from build123d import *
from OCP.BRepFilletAPI import BRepFilletAPI_MakeChamfer

# Parameters (mm, degrees)
SKETCH1_W           = 16
SKETCH1_H           = 16
BOSS_EXTRUDE1_DEPTH = 25
CIRPATTERN1_COUNT   = 5
CIRPATTERN1_ANGLE   = 160
CHAMFER1_SIZE       = 15
CHAMFER1_SIZE2      = 8.660254038
CHAMFER3_SIZE       = 10
CHAMFER3_SIZE_2     = 5.773502692


with BuildPart() as part:
    # Sketch1 → Boss-Extrude1 (new body)
    with BuildSketch(Plane.XY):
        with BuildLine():
            Line((-150, 0), (0, 0))
            ThreePointArc((0, 0), (-75, -75), (-150, 0))
        make_face()
        with Locations((-55.5, -23)):
            Rectangle(SKETCH1_W, SKETCH1_H, mode=Mode.SUBTRACT)
        with Locations((-94.5, -23)):
            Rectangle(SKETCH1_W, SKETCH1_H, mode=Mode.SUBTRACT)
    extrude(amount=BOSS_EXTRUDE1_DEPTH)

    # Sketch4 → Ø4.0mm Dowel Hole2 (revolve, cut)
    with BuildSketch(Plane(origin=(-1.139418524, -13.023613325, 12.5), x_dir=(0.17364817766693047, 0.9848077530122081, 0), z_dir=(0, 0, 1))):
        Polygon((0, 0), (0, 17.201721238), (2, 16), (2, 0.025), (2.025, 0), align=None)
    f_4_0mm_dowel_hole2 = revolve(axis=Axis((5.114110708, -14.126279253, 12.5), (-0.9848077530122081, 0.17364817766693044, 0)), mode=Mode.SUBTRACT)

    # CirPattern1: Ø4.0mm Dowel Hole2 ×5 about axis
    cirpattern1_axis = Axis((-75, 0, 0), (0, 0, -1))
    for i in range(1, CIRPATTERN1_COUNT):
        add(f_4_0mm_dowel_hole2.rotate(cirpattern1_axis, i * CIRPATTERN1_ANGLE / (CIRPATTERN1_COUNT - 1)), mode=Mode.SUBTRACT)

    # Chamfer1: one chamfer whose edges measure the first distance from different faces: ONE call of the kernel's chamfer builder (chamfer() names one face for all edges)
    chamfer1_edges_1 = [part.edges().sort_by_distance(p)[0] for p in [
        (-55.5, -15, 0),
    ]]
    chamfer1_side_1 = [part.faces().sort_by_distance(p)[0] for p in [
        (-55.5, -15, 12.5),
    ]]
    chamfer1_edges_2 = [part.edges().sort_by_distance(p)[0] for p in [
        (-94.5, -15, 0),
    ]]
    chamfer1_side_2 = [part.faces().sort_by_distance(p)[0] for p in [
        (-94.5, -15, 12.5),
    ]]
    chamfer1 = BRepFilletAPI_MakeChamfer(part.part.solid().wrapped)
    for e in chamfer1_edges_1:
        chamfer1.Add(CHAMFER1_SIZE, CHAMFER1_SIZE2, e.wrapped, chamfer1_side_1[0].wrapped)  # the first distance lies on this face
    for e in chamfer1_edges_2:
        chamfer1.Add(CHAMFER1_SIZE, CHAMFER1_SIZE2, e.wrapped, chamfer1_side_2[0].wrapped)  # the first distance lies on this face
    add(Compound.cast(chamfer1.Shape()), mode=Mode.REPLACE)

    # Chamfer3
    chamfer3_edges_1 = [part.edges().sort_by_distance(p)[0] for p in [
        (-102.5, -23, 25),
    ]]
    chamfer3_side_1 = [part.faces().sort_by_distance(p)[0] for p in [
        (-102.5, -23, 24.884529946),
    ]]
    chamfer3_edges_2 = [part.edges().sort_by_distance(p)[0] for p in [
        (-94.5, -15, 25),
    ]]
    chamfer3_side_2 = [part.faces().sort_by_distance(p)[0] for p in [
        (-94.5, -14.884529946, 25),
    ]]
    chamfer3_edges_3 = [part.edges().sort_by_distance(p)[0] for p in [
        (-86.5, -23, 25),
    ]]
    chamfer3_side_3 = [part.faces().sort_by_distance(p)[0] for p in [
        (-86.5, -23, 24.884529946),
    ]]
    chamfer3_edges_4 = [part.edges().sort_by_distance(p)[0] for p in [
        (-47.5, -23, 25),
    ]]
    chamfer3_side_4 = [part.faces().sort_by_distance(p)[0] for p in [
        (-47.5, -23, 24.884529946),
    ]]
    chamfer3_edges_5 = [part.edges().sort_by_distance(p)[0] for p in [
        (-55.5, -15, 25),
    ]]
    chamfer3_side_5 = [part.faces().sort_by_distance(p)[0] for p in [
        (-55.5, -15, 24.884529946),
    ]]
    chamfer3_edges_6 = [part.edges().sort_by_distance(p)[0] for p in [
        (-63.5, -23, 25),
    ]]
    chamfer3_side_6 = [part.faces().sort_by_distance(p)[0] for p in [
        (-63.5, -23, 24.884529946),
    ]]
    chamfer3 = BRepFilletAPI_MakeChamfer(part.part.solid().wrapped)
    for e in chamfer3_edges_1:
        chamfer3.Add(CHAMFER3_SIZE - 0.0001, CHAMFER3_SIZE_2 - 0.0001, e.wrapped, chamfer3_side_1[0].wrapped)
    for e in chamfer3_edges_2:
        chamfer3.Add(CHAMFER3_SIZE_2 - 0.0001, CHAMFER3_SIZE - 0.0001, e.wrapped, chamfer3_side_2[0].wrapped)
    for e in chamfer3_edges_3:
        chamfer3.Add(CHAMFER3_SIZE - 0.0001, CHAMFER3_SIZE_2 - 0.0001, e.wrapped, chamfer3_side_3[0].wrapped)
    for e in chamfer3_edges_4:
        chamfer3.Add(CHAMFER3_SIZE - 0.0001, CHAMFER3_SIZE_2 - 0.0001, e.wrapped, chamfer3_side_4[0].wrapped)
    for e in chamfer3_edges_5:
        chamfer3.Add(CHAMFER3_SIZE - 0.0001, CHAMFER3_SIZE_2 - 0.0001, e.wrapped, chamfer3_side_5[0].wrapped)
    for e in chamfer3_edges_6:
        chamfer3.Add(CHAMFER3_SIZE - 0.0001, CHAMFER3_SIZE_2 - 0.0001, e.wrapped, chamfer3_side_6[0].wrapped)
    add(Compound.cast(chamfer3.Shape()), mode=Mode.REPLACE)  # a hair under: the kernel refuses the full size


solid = part.part
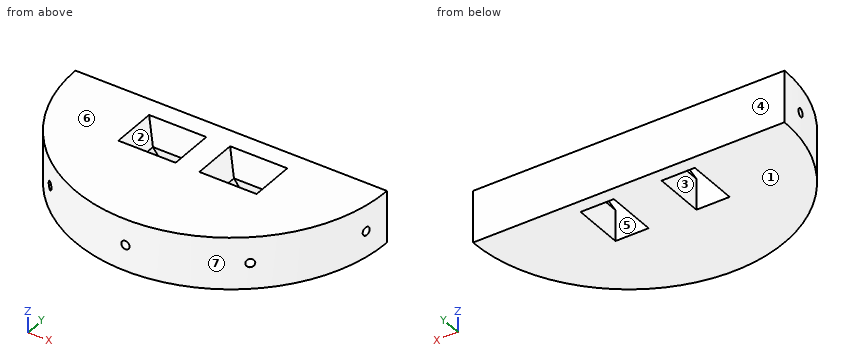
The model under review builds one solid part; all positions refer to its coordinate system, in mm. Face numbers are marked on the shaded views. A direction names the side the tool comes from. Give positions to 0.01 mm unless a question says otherwise; leave off trailing zeros. Write each loop counter-clockwise with the first axis right and the second up, starting at its lowest first coordinate (ties: lowest second). Pieces come first, ordered by that corner, then holes.
1. Wall thickness on L1, parallel to Z at x = -75, y = -71; L2, parallel to Y at x = -120, z = 13.5; L3, parallel to Y at x = -91.5, z = 2.5: over which ranges is each line inside the solid? List them lowest first.
2. Add section B-B, the plane z = 7.5. Write out the cut boundary in (x, y).
3. Tool access review of the marked faces 1, 2 and 3: name each direction out of +Z, -Z, +X, -X, +Y, -Y from which nothing blocks a thin tool from reaching the whole face with its end or side.
4. Draft analysis for pull direction Y (two halves, no side actions). For the marked faces 4, 5, 6 and 7, state which applies: +Y half, -Y half, draft (parallel to the pull), parting line (faces both ways), or undercut.
5. Add section C-C, the plane y = -25. Write out the cut boundary in (x, z).
6. Add section D-D, the plane x = -65. Write out the cut boundary in (y, z).
7. For P1, Ø12, axis at y = -42, z = 3, coming from the +X side; P2, Ø3, axis at y = -51, z = 6, coming from the +X side; P3, Ø2, axis at y = -62.5, z = 6.5, coming from the +X side; P4, Ø4.5, axis at x = -75, z = 12.5, coming from the -Y side, all flat-tipped, find the tip position at first contact; note any pin that passes through.
Worked answers:
1. L1: z = 0 to 10.5, 14.5 to 25
1. L2: y = -60 to -56.32, -50.93 to 0
1. L3: y = -73.16 to -31, -7.78 to 0
2. outline: (-150, 0) arc R75 ccw to (0, 0) - close; hole (-102.5, -31) - (-86.5, -31) - (-86.5, -10.67) - (-102.5, -10.67) - close; hole (-63.5, -31) - (-47.5, -31) - (-47.5, -10.67) - (-63.5, -10.67) - close
3. face 1: -Z, +X, -X, +Y, -Y
3. face 2: +Z
3. face 3: -Z
4. face 4: +Y half
4. face 5: undercut
4. face 6: draft
4. face 7: -Y half
5. outline: (-145.71, 0) - (-102.5, 0) - (-102.5, 15) - (-108.27, 25) - (-145.71, 25) - close; (-86.5, 0) - (-63.5, 0) - (-63.5, 15) - (-69.27, 25) - (-80.73, 25) - (-86.5, 15) - close; (-47.5, 0) - (-4.29, 0) - (-4.29, 25) - (-41.73, 25) - (-47.5, 15) - close
6. outline: (-74.33, 0) - (0, 0) - (0, 25) - (-9.23, 25) - (-13.5, 17.6) - (-31, 17.6) - (-31, 25) - (-74.33, 25) - close
7. P1: stops at x = -9.2
7. P2: stops at x = -18.66
7. P3: stops at x = -32.07
7. P4: stops at y = -75
